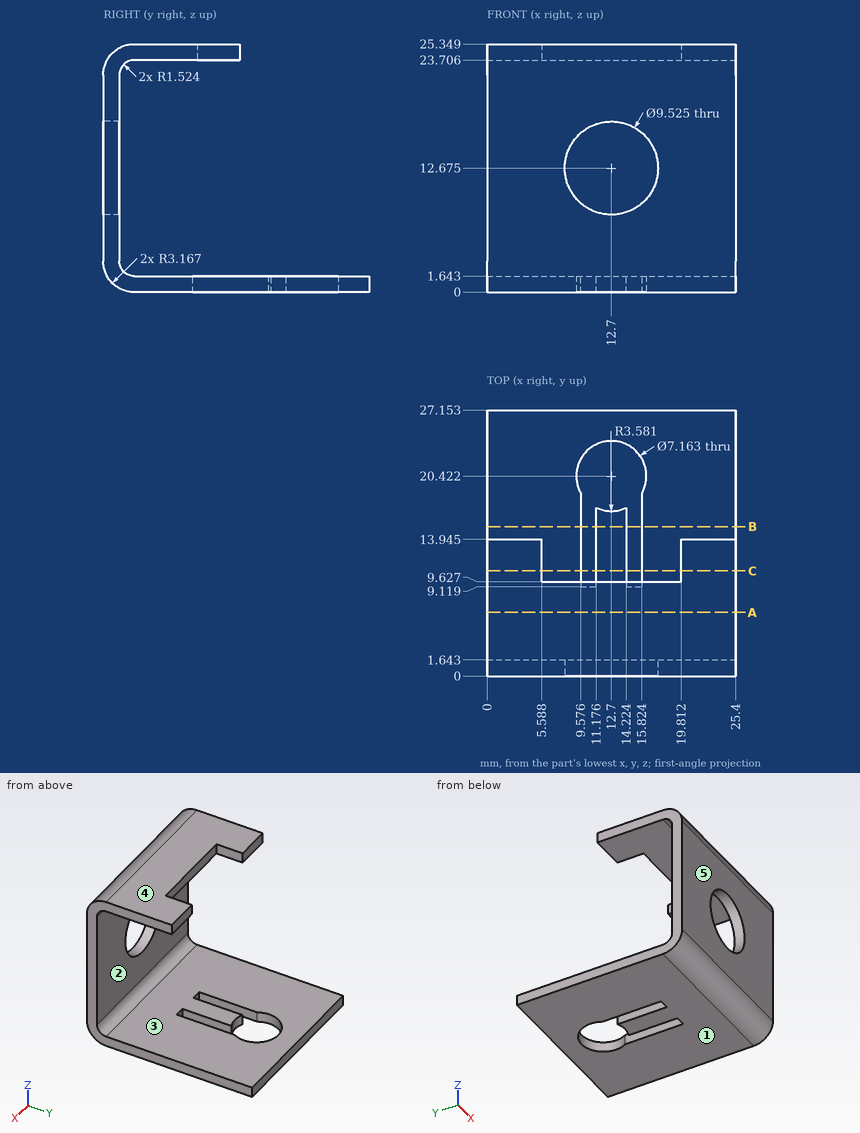
The drawing under review shows one solid part. Ordinate dimensions are in mm from its lowest x, y, z. A direction names the side the tool comes from. Coordinates: 2 decimals unless noted, no trailing zeros. Order: outer loops, then holes, each group sorted by start corner. A loop starts at its lowest first (then second) coordinate and runs counter-clockwise, first axis right, second up. Notation, with made-up numbers: (47, -32) -> (76, -32) arc R31 ccw to (76, 4) -> close; hole circle Ø7 at (78, 81.25). An arc over 180 degrees is marked (long way). Answer in a Markdown table with one row per item. Add a question column.
Item 1: We need section C-C on y = 10.75. Give the number of separate pieces and of enclosed holes in the cut face.
Item 2: Mouldability with a two-part tool opening along Z and no side actions: class the marked faces 3, 4 and 5 as +Z half, -Z half, draft (parallel to the pull), parting line (faces both ways), or undercut.
Item 3: We need section A-A on y = 6.5. Write out the cut boundary in (x, z).
Item 4: Clearance check with flat-ended pins moving along their axes: pin 1 (9.5 mm diameter, centred on x = 9, z = 11, fed in from +Y); pin 2 (1.8 mm diameter, centred on x = 22, z = 24.5, fed in from +Y) (1 decimal); pin 3 (0.5 mm diameter, centred on x = 15, z = 25, fed in from +Y). State where each tip first meets the part, or that it passes through.
Item 5: We need section B-B on y = 15.25. Write out the cut boundary in (x, z) (1 decimal).
Item 6: Machinability: for the marked faces 1 and 2, which of the approach directions +Z, -Z, +X, -X, +Y, -Y give a long, thin tool a straight path to every point of the face, cutting with its end or side? Answer none if there is none.
Item 7: To check wall thickness, follow probe 1 along Z at (x, y) = (14.75, 5.25); probe 2 along X at (y, z) = (13, 24.25); probe 3 along Z at (x, y) = (12.7, 0.6) (1 decimal). State the ranges of each line that lie inside material, in increasing order.
Final values:
| question | item | result |
|---|---|---|
| 1 | separate pieces | 5 |
| 1 | enclosed holes | 0 |
| 2 | face 3 | undercut |
| 2 | face 4 | +Z half |
| 2 | face 5 | draft |
| 3 | outline | (0, 0) -> (25.4, 0) -> (25.4, 1.64) -> (0, 1.64) -> close; (0, 23.71) -> (25.4, 23.71) -> (25.4, 25.35) -> (0, 25.35) -> close |
| 4 | pin 1 | stops at y = 1.64 |
| 4 | pin 2 | stops at y = 13.9 |
| 4 | pin 3 | stops at y = 9.63 |
| 5 | outline | (0, 0) -> (9.6, 0) -> (9.6, 1.6) -> (0, 1.6) -> close; (11.2, 0) -> (14.2, 0) -> (14.2, 1.6) -> (11.2, 1.6) -> close; (15.8, 0) -> (25.4, 0) -> (25.4, 1.6) -> (15.8, 1.6) -> close |
| 6 | face 1 | -Z, +X, -X, +Y, -Y |
| 6 | face 2 | +X, -X, +Y |
| 7 | probe 1 | z = 0 to 1.64, 23.71 to 25.35 |
| 7 | probe 2 | x = 0 to 5.59, 19.81 to 25.4 |
| 7 | probe 3 | z = 1.3 to 7.9, 17.4 to 24 |
